For this review, take the finished solid that the model builds, in its own axes (mm). Coordinates: 2 decimals unless noted, no trailing zeros. Loops run counter-clockwise (first coordinate to the right, second up) from the corner with the lowest first, then second, coordinate; pieces in that order, holes last. Notation, with made-up numbers: (-7, 54.25) -> (30, 54.25) arc R24 ccw to (30, 85.25) -> close; hole circle Ø3 at (29, 26). An arc over 180 degrees is marked (long way). One line per item, written item: value.
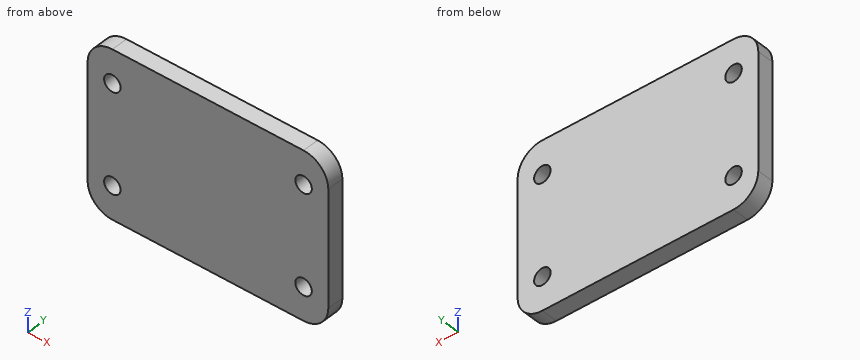
from build123d import *

# Parameters (mm, degrees)
SALIENTE_EXTRUIR1_DEPTH  = 10
CROQUIS2_R               = 5
CORTAR_EXTRUIR1_DEPTH    = 10
MATRIZL1_COUNT           = 3
MATRIZL1_PITCH           = 116
MATRIZL2_COUNT           = 3
MATRIZL2_PITCH           = 60
MATRIZL2_COPY_1_SKETCH_R = 5
MATRIZL2_COPY_1_DEPTH    = 10
MATRIZL2_COPY_2_SKETCH_R = 5
MATRIZL2_COPY_2_DEPTH    = 10
MATRIZL2_COPY_3_SKETCH_R = 5
MATRIZL2_COPY_3_DEPTH    = 10
MATRIZL2_COPY_4_SKETCH_R = 5
MATRIZL2_COPY_4_DEPTH    = 10


with BuildPart() as part:
    # Croquis1 → Saliente-Extruir1 (new body)
    with BuildSketch(Plane(origin=(0, 0, 0), x_dir=(1, 0, 0), z_dir=(0, 1, 0))):
        with BuildLine():
            Line((58, -50), (-58, -50))
            ThreePointArc((-58, -50), (-68.606601718, -45.606601718), (-73, -35))
            Line((-73, -35), (-73, 35))
            ThreePointArc((-73, 35), (-68.606601718, 45.606601718), (-58, 50))
            Line((-58, 50), (58, 50))
            ThreePointArc((58, 50), (68.606601718, 45.606601718), (73, 35))
            Line((73, 35), (73, -35))
            ThreePointArc((73, -35), (68.606601718, -45.606601718), (58, -50))
        make_face()
    extrude(amount=SALIENTE_EXTRUIR1_DEPTH)

    # Croquis2 → Cortar-Extruir1 (cut)
    with BuildSketch(Plane(origin=(0, 10, 0), x_dir=(1, 0, 0), z_dir=(0, 1, 0))):
        with Locations(Location((-58, 30, 0), (0, 0, 270))):
            Circle(CROQUIS2_R)
    cortar_extruir1 = extrude(amount=-CORTAR_EXTRUIR1_DEPTH, mode=Mode.SUBTRACT)

    # MatrizL1: Cortar-Extruir1 ×3
    with Locations(*[(i * MATRIZL1_PITCH, 0, 0) for i in range(1, MATRIZL1_COUNT)]):
        add(cortar_extruir1, mode=Mode.SUBTRACT)

    # MatrizL2: Cortar-Extruir1 ×3
    with Locations(*[(0, 0, i * MATRIZL2_PITCH) for i in range(1, MATRIZL2_COUNT)]):
        add(cortar_extruir1, mode=Mode.SUBTRACT)

    # MatrizL2 copy 1 sketch → MatrizL2 copy 1 (cut)
    with BuildSketch(Plane(origin=(116, 10, 60), x_dir=(1, 0, 0), z_dir=(0, 1, 0))):
        with Locations(Location((-58, 30, 0), (0, 0, 270))):
            Circle(MATRIZL2_COPY_1_SKETCH_R)
    extrude(amount=-MATRIZL2_COPY_1_DEPTH, mode=Mode.SUBTRACT)

    # MatrizL2 copy 2 sketch → MatrizL2 copy 2 (cut)
    with BuildSketch(Plane(origin=(116, 10, 120), x_dir=(1, 0, 0), z_dir=(0, 1, 0))):
        with Locations(Location((-58, 30, 0), (0, 0, 270))):
            Circle(MATRIZL2_COPY_2_SKETCH_R)
    extrude(amount=-MATRIZL2_COPY_2_DEPTH, mode=Mode.SUBTRACT)

    # MatrizL2 copy 3 sketch → MatrizL2 copy 3 (cut)
    with BuildSketch(Plane(origin=(232, 10, 60), x_dir=(1, 0, 0), z_dir=(0, 1, 0))):
        with Locations(Location((-58, 30, 0), (0, 0, 270))):
            Circle(MATRIZL2_COPY_3_SKETCH_R)
    extrude(amount=-MATRIZL2_COPY_3_DEPTH, mode=Mode.SUBTRACT)

    # MatrizL2 copy 4 sketch → MatrizL2 copy 4 (cut)
    with BuildSketch(Plane(origin=(232, 10, 120), x_dir=(1, 0, 0), z_dir=(0, 1, 0))):
        with Locations(Location((-58, 30, 0), (0, 0, 270))):
            Circle(MATRIZL2_COPY_4_SKETCH_R)
    extrude(amount=-MATRIZL2_COPY_4_DEPTH, mode=Mode.SUBTRACT)


solid = part.part
1. Take a section at A-A, the plane z = -30. Give the boundary of the cut face in (x, y), and give its area (3 significant figures).
Return value:
outline: (-73, 0) -> (-63, 0) -> (-63, 10) -> (-73, 10) -> close; (-53, 0) -> (53, 0) -> (53, 10) -> (-53, 10) -> close; (63, 0) -> (73, 0) -> (73, 10) -> (63, 10) -> close
area: 1,260 mm2
2. Take a section at B-B, the plane y = 5.5. Give the boundary of the cut face in (x, z), and give its area (3 significant figures).
Return value:
outline: (-73, -35) arc R15 ccw to (-58, -50) -> (58, -50) arc R15 ccw to (73, -35) -> (73, 35) arc R15 ccw to (58, 50) -> (-58, 50) arc R15 ccw to (-73, 35) -> close; hole circle Ø10 at (-58, -30); hole circle Ø10 at (-58, 30); hole circle Ø10 at (58, -30); hole circle Ø10 at (58, 30)
area: 14,100 mm2
3. To check wall thickness, follow probe 1 along X at (y, z) = (6, -30); probe 2 along Z at (x, y) = (59, 0.5); probe 3 along X at (y, z) = (1.25, 33). State the ranges of each line that lie inside material, in increasing order. Write a range as from..to.
Return value:
probe 1: x = -73..-63, -53..53, 63..73
probe 2: z = -49.97..-34.9, -25.1..25.1, 34.9..49.97
probe 3: x = -73..-62, -54..54, 62..73
